The listing builds one solid part. Answer for the finished solid, in the listing's coordinates (mm). Face numbers are marked on the shaded views. A direction names the side the tool comes from. Round coordinates to 2 decimals unless told otherwise and drop trailing zeros. Write each loop counter-clockwise with the first axis right and the second up, starting at its lowest first coordinate (ties: lowest second). Pieces come first, ordered by that corner, then holes.
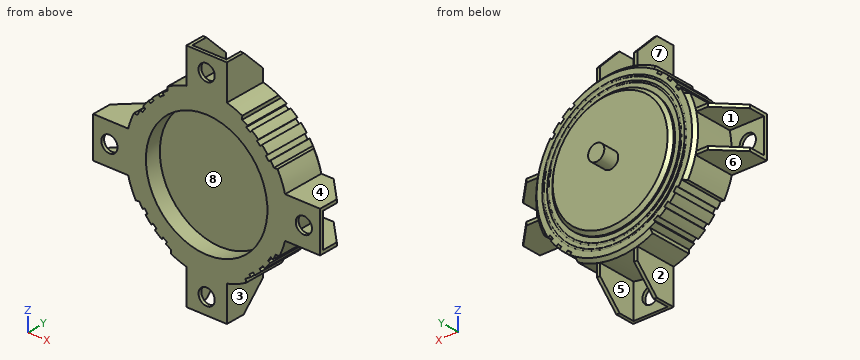
from build123d import *

# Parameters (mm, degrees)
CHAMFER1_SIZE                   = 2
BOSS_EXTRUDE1_DEPTH             = 70
CHAMFER2_SIZE                   = 14
SKETCH3_R                       = 5
CUT_EXTRUDE1_DEPTH              = 70
CIRPATTERN1_COUNT               = 4
CHAMFER2_OF_CIRPATTERN1_SIZE    = 14
CUT_EXTRUDE2_START              = 70
CUT_EXTRUDE2_DEPTH              = 70
CUT_EXTRUDE3_DEPTH              = 70
CIRPATTERN2_COUNT               = 2
CIRPATTERN2_ANGLE               = 10
CIRPATTERN2_THE_OTHER_WAY_COUNT = 2
CIRPATTERN2_THE_OTHER_WAY_ANGLE = 10
CIRPATTERN3_COUNT               = 4
CIRPATTERN3_COPY_1_DEPTH        = 70
CIRPATTERN3_COPY_2_DEPTH        = 70
CIRPATTERN3_COPY_3_DEPTH        = 70
CIRPATTERN3_COPY_4_DEPTH        = 70
CIRPATTERN3_COPY_5_DEPTH        = 70
CIRPATTERN3_COPY_6_DEPTH        = 70
CUT_SWEEP1_PROFILE_R            = 0.5
CUT_SWEEP2_PROFILE_R            = 0.5
CUT_EXTRUDE4_START              = -10
SKETCH16_R                      = 37.5
CUT_EXTRUDE4_DEPTH              = 10


with BuildPart() as part:
    # Sketch1 → Revolve1 (revolve)
    with BuildSketch(Plane.XY, mode=Mode.PRIVATE) as revolve1_sk:
        Polygon((0, 0), (-50, 0), (-50, 28), (-37.5, 28), (-37.5, 31), (-5, 31), (-5, 41), (0, 41), align=None)
    revolve(revolve1_sk.sketch.rotate(Axis((0, 0, 0), (0, 1, 0)), 270), axis=Axis((0, 0, 0), (0, 1, 0)))

    # Chamfer1
    chamfer1_edges = [part.edges().sort_by_distance(p)[0] for p in [
        (0, 31, 37.5),
        (0, 28, 50),
    ]]
    chamfer(chamfer1_edges, length=CHAMFER1_SIZE)

    # Sketch2 → Boss-Extrude1 (add)
    with BuildSketch(Plane.XY):
        Polygon((-12.5, 26), (-12.5, 0), (12.5, 0), (12.5, 26), (10.5, 26), (10.5, 2), (-10.5, 2), (-10.5, 26), align=None)
    boss_extrude1 = extrude(amount=BOSS_EXTRUDE1_DEPTH)

    # Chamfer2
    chamfer2_edges = [part.edges().sort_by_distance(p)[0] for p in [
        (-11.5, 26, 70),
        (11.5, 26, 70),
    ]]
    chamfer(chamfer2_edges, length=CHAMFER2_SIZE)

    # Sketch3 → Cut-Extrude1 (cut)
    with BuildSketch(Plane(origin=(0, 0, 0), x_dir=(1, 0, 0), z_dir=(0, 1, 0))):
        with Locations(Location((0, -60, 0), (0, 0, 90))):
            Circle(SKETCH3_R)
    cut_extrude1 = extrude(amount=CUT_EXTRUDE1_DEPTH, mode=Mode.SUBTRACT)

    # CirPattern1: Boss-Extrude1, Cut-Extrude1 ×4 about axis
    cirpattern1_axis = Axis((0, 0, 0), (0, 1, 0))
    add([boss_extrude1.rotate(cirpattern1_axis, i * 360 / CIRPATTERN1_COUNT) for i in range(1, CIRPATTERN1_COUNT)])
    add([cut_extrude1.rotate(cirpattern1_axis, i * 360 / CIRPATTERN1_COUNT) for i in range(1, CIRPATTERN1_COUNT)], mode=Mode.SUBTRACT)

    # Chamfer2 of CirPattern1
    chamfer2_of_cirpattern1_edges = [part.edges().sort_by_distance(p)[0] for p in [
        (70, 26, 11.5),
        (70, 26, -11.5),
        (11.5, 26, -70),
        (-11.5, 26, -70),
        (-70, 26, -11.5),
        (-70, 26, 11.5),
    ]]
    chamfer(chamfer2_of_cirpattern1_edges, length=CHAMFER2_OF_CIRPATTERN1_SIZE)

    # Sketch4 → Cut-Extrude2 (cut)
    with BuildSketch(Plane(origin=(0, 0, 0), x_dir=(1, 0, 0), z_dir=(0, 1, 0)).offset(CUT_EXTRUDE2_START)):
        with BuildLine():
            Line((21.951196001, -42.686590332), (21.990145173, -44.904715958))
            ThreePointArc((21.990145173, -44.904715958), (34.448676313, -36.239325329), (43.73374037, -24.23551017))
            Line((43.73374037, -24.23551017), (41.520431678, -24.084305123))
            ThreePointArc((41.520431678, -24.084305123), (33.07072926, -34.789752316), (21.951196001, -42.686590332))
        make_face()
    cut_extrude2 = extrude(amount=-CUT_EXTRUDE2_DEPTH, mode=Mode.SUBTRACT)

    # Sketch5 → Cut-Extrude3 (cut)
    with BuildSketch(Plane(origin=(0, 0, 0), x_dir=(1, 0, 0), z_dir=(0, 1, 0))):
        Polygon((33.01700979, -36.910392365), (35.191369309, -34.843471786), (33.124448731, -32.669112267), (30.950089211, -34.736032845), align=None)
    cut_extrude3 = extrude(amount=CUT_EXTRUDE3_DEPTH, mode=Mode.SUBTRACT)

    # CirPattern2: Cut-Extrude3 ×2 about axis
    cirpattern2_axis = Axis((0, 0, 0), (0, 1, 0))
    for i in range(1, CIRPATTERN2_COUNT):
        add(cut_extrude3.rotate(cirpattern2_axis, i * CIRPATTERN2_ANGLE / (CIRPATTERN2_COUNT - 1)), mode=Mode.SUBTRACT)

    # CirPattern2 the other way: Cut-Extrude3 ×2 about axis
    cirpattern2_the_other_way_axis = Axis((0, 0, 0), (0, -1, 0))
    for i in range(1, CIRPATTERN2_THE_OTHER_WAY_COUNT):
        add(cut_extrude3.rotate(cirpattern2_the_other_way_axis, i * CIRPATTERN2_THE_OTHER_WAY_ANGLE / (CIRPATTERN2_THE_OTHER_WAY_COUNT - 1)), mode=Mode.SUBTRACT)

    # CirPattern3: Cut-Extrude2, Cut-Extrude3 ×4 about axis
    cirpattern3_axis = Axis((0, 0, 0), (0, 1, 0))
    add([cut_extrude2.rotate(cirpattern3_axis, i * 360 / CIRPATTERN3_COUNT) for i in range(1, CIRPATTERN3_COUNT)], mode=Mode.SUBTRACT)
    add([cut_extrude3.rotate(cirpattern3_axis, i * 360 / CIRPATTERN3_COUNT) for i in range(1, CIRPATTERN3_COUNT)], mode=Mode.SUBTRACT)

    # CirPattern3 copy 1 sketch → CirPattern3 copy 1 (cut)
    with BuildSketch(Plane(origin=(0, 0, 0), x_dir=(-0.17364817766693091, 0, -0.9848077530122079), z_dir=(0, 1, 0))):
        Polygon((33.01700979, -36.910392365), (35.191369309, -34.843471786), (33.124448731, -32.669112267), (30.950089211, -34.736032845), align=None)
    extrude(amount=CIRPATTERN3_COPY_1_DEPTH, mode=Mode.SUBTRACT)

    # CirPattern3 copy 2 sketch → CirPattern3 copy 2 (cut)
    with BuildSketch(Plane(origin=(0, 0, 0), x_dir=(-0.9848077530122079, 0, 0.17364817766693086), z_dir=(0, 1, 0))):
        Polygon((33.01700979, -36.910392365), (35.191369309, -34.843471786), (33.124448731, -32.669112267), (30.950089211, -34.736032845), align=None)
    extrude(amount=CIRPATTERN3_COPY_2_DEPTH, mode=Mode.SUBTRACT)

    # CirPattern3 copy 3 sketch → CirPattern3 copy 3 (cut)
    with BuildSketch(Plane(origin=(0, 0, 0), x_dir=(0.17364817766693078, 0, 0.9848077530122079), z_dir=(0, 1, 0))):
        Polygon((33.01700979, -36.910392365), (35.191369309, -34.843471786), (33.124448731, -32.669112267), (30.950089211, -34.736032845), align=None)
    extrude(amount=CIRPATTERN3_COPY_3_DEPTH, mode=Mode.SUBTRACT)

    # CirPattern3 copy 4 sketch → CirPattern3 copy 4 (cut)
    with BuildSketch(Plane(origin=(0, 0, 0), x_dir=(0.17364817766693103, 0, -0.9848077530122079), z_dir=(0, 1, 0))):
        Polygon((33.01700979, -36.910392365), (35.191369309, -34.843471786), (33.124448731, -32.669112267), (30.950089211, -34.736032845), align=None)
    extrude(amount=CIRPATTERN3_COPY_4_DEPTH, mode=Mode.SUBTRACT)

    # CirPattern3 copy 5 sketch → CirPattern3 copy 5 (cut)
    with BuildSketch(Plane(origin=(0, 0, 0), x_dir=(-0.9848077530122079, 0, -0.17364817766693108), z_dir=(0, 1, 0))):
        Polygon((33.01700979, -36.910392365), (35.191369309, -34.843471786), (33.124448731, -32.669112267), (30.950089211, -34.736032845), align=None)
    extrude(amount=CIRPATTERN3_COPY_5_DEPTH, mode=Mode.SUBTRACT)

    # CirPattern3 copy 6 sketch → CirPattern3 copy 6 (cut)
    with BuildSketch(Plane(origin=(0, 0, 0), x_dir=(-0.17364817766693116, 0, 0.9848077530122079), z_dir=(0, 1, 0))):
        Polygon((33.01700979, -36.910392365), (35.191369309, -34.843471786), (33.124448731, -32.669112267), (30.950089211, -34.736032845), align=None)
    extrude(amount=CIRPATTERN3_COPY_6_DEPTH, mode=Mode.SUBTRACT)

    # Cut-Sweep1: sweep along a path in Sketch6
    with BuildLine(Plane(origin=(0, 28, 0), x_dir=(1, 0, 0), z_dir=(0, 1, 0))) as cut_sweep1_path:
        CenterArc((0, 0), 41, 0, 360)
    # Cut-Sweep1 profile (on start of the path) → Cut-Sweep1 (sweep, cut)
    with BuildSketch(Plane(origin=(41, 28, 0), x_dir=(-1, 0, 0), z_dir=(0, 0, -1))):
        Circle(CUT_SWEEP1_PROFILE_R)
    sweep(path=cut_sweep1_path.line, mode=Mode.SUBTRACT)

    # Cut-Sweep2: sweep along a path in Sketch7
    with BuildLine(Plane(origin=(0, 28, 0), x_dir=(1, 0, 0), z_dir=(0, 1, 0))) as cut_sweep2_path:
        CenterArc((0, 0), 44, 0, 360)
    # Cut-Sweep2 profile (on start of the path) → Cut-Sweep2 (sweep, cut)
    with BuildSketch(Plane(origin=(44, 28, 0), x_dir=(-1, 0, 0), z_dir=(0, 0, -1))):
        Circle(CUT_SWEEP2_PROFILE_R)
    sweep(path=cut_sweep2_path.line, mode=Mode.SUBTRACT)

    # Sketch16 → Cut-Extrude4 (cut)
    with BuildSketch(Plane.XZ.offset(CUT_EXTRUDE4_START)):
        with Locations(Location((0, 0, 0), (0, 0, 270))):
            Circle(SKETCH16_R)
    extrude(amount=CUT_EXTRUDE4_DEPTH, mode=Mode.SUBTRACT)


solid = part.part
1. Section C-C on x = 0 is taken. Give the number of separate pieces and of enclosed holes in the cut face, plus the area to 3 significant figures.
Geometry says:
separate pieces: 3
enclosed holes: 0
area: 2,410 mm2
2. Given pin 1 (3 mm diameter, centred on x = -11, z = 6, fed in from -Y); pin 2 (6.5 mm diameter, centred on x = -56, y = 9, fed in from -Z); pin 3 (17 mm diameter, centred on y = 12.5, z = -57, fed in from -X); pin 4 (12 mm diameter, centred on x = -53.5, z = -20.5, fed in from -Y), each flat-ended and moving along its own axis, determine where each tip first touches the part or whether it passes through.
Geometry says:
pin 1: stops at y = 10
pin 2: stops at z = -12.5
pin 3: stops at x = -12.5
pin 4: passes through
3. Section B-B on z = -60 is taken. Determine the outline of the cut face in (x, y), plus the area to 3 significant figures.
Geometry says:
outline: (-12.5, 0) - (-5, 0) - (-5, 2) - (-10.5, 2) - (-10.5, 22) - (-12.5, 22) - close; (5, 0) - (12.5, 0) - (12.5, 22) - (10.5, 22) - (10.5, 2) - (5, 2) - close
area: 110 mm2
4. Straight lines are drawn through the part: line 1 along X through (y, z) = (19.5, 56); line 2 along X through (y, z) = (1, -60). For each, find the intervals that lie inside material, in ascending order.
Geometry says:
line 1: x = -12.5 to -10.5, 10.5 to 12.5
line 2: x = -12.5 to -5, 5 to 12.5
5. For a pull along Z with two mould halves and no side action, classify the marked faces 6, 7 and 8 as released by +Z, released by -Z, zero draft, split by the parting line, or undercut.
Geometry says:
face 6: released by -Z
face 7: zero draft
face 8: undercut
6. Section D-D on y = 38 is taken. Determine the outline of the cut face in (x, z).
Geometry says:
outline: circle Ø10 at (0, 0)
7. Section A-A on x = -60 is taken. Determine the outline of the cut face in (y, z).
Geometry says:
outline: (0, -12.5) - (22, -12.5) - (22, -10.5) - (2, -10.5) - (2, -5) - (0, -5) - close; (0, 5) - (2, 5) - (2, 10.5) - (22, 10.5) - (22, 12.5) - (0, 12.5) - close
8. A tool of negligible diameter and unlimited length cuts with its end or side. For the marked faces 1, 2, 3, 4 and 5, from which of +Z, -Z, +X, -X, +Y, -Y can it reach the whole face along a straight path? Write none if from no direction.
Geometry says:
face 1: -X, +Y
face 2: -Z, -X, +Y, -Y
face 3: -Z, +X, +Y, -Y
face 4: +Z, +X, +Y, -Y
face 5: -Z, +Y
